from build123d import *

# Parameters (mm, degrees)
SKETCH1_W           = 79.816604327
SKETCH1_H           = 61.580684207
BOSS_EXTRUDE1_DEPTH = 20
CUT_EXTRUDE1_START  = -18.943875
SKETCH3_R           = 4
CUT_EXTRUDE1_DEPTH  = 80.816604514


with BuildPart() as part:
    # Sketch1 → Boss-Extrude1 (new body)
    with BuildSketch(Plane.XY):
        with Locations((-58.852177351, -19.652156424)):
            Rectangle(SKETCH1_W, SKETCH1_H)
    extrude(amount=BOSS_EXTRUDE1_DEPTH)

    # Sketch3 → Cut-Extrude1 (cut, through all)
    with BuildSketch(Plane(origin=(0, 0, 0), x_dir=(0, 0, -1), z_dir=(1, 0, 0)).offset(CUT_EXTRUDE1_START)):
        with Locations((-10, -5.101602078)):
            Circle(SKETCH3_R)
    extrude(amount=-CUT_EXTRUDE1_DEPTH, mode=Mode.SUBTRACT)


solid = part.part
Design review of the part built by this model. Coordinates are the model's own, in mm. Give positions to 0.01 mm unless a question says otherwise; leave off trailing zeros. Write each loop counter-clockwise with the first axis right and the second up, starting at its lowest first coordinate (ties: lowest second). Pieces come first, ordered by that corner, then holes. Notation, with made-up numbers: M -36,21 L -3,21 A12 cw -3,29 Z; hole C -24.75,-16.75 d11. An arc over 180 degrees is marked long. Return JSON: item names as keys, results as strings. Group by question number.
Item 1: Take a section at A-A (z = 10). Give the boundary of the cut face in (x, y), plus the area to 3 significant figures.
Item 2: Take a section at B-B (x = -44). Give the boundary of the cut face in (y, z), plus the area to 3 significant figures.
Item 3: The part is to be moulded in two halves that separate along Y. For faces 1 (the flat face through (-59, -19, 20)), 2 (the flat face through (-59, -50.442, 10)), 3 (the cylindrical face through (-58.3, -9, 10.9)), say which applies: pulls with the +Y half, pulls with the -Y half, needs draft (parallel to the pull), parting line crosses it, or undercut.
Item 4: Wall thickness on line 1 along Y through (x, z) = (-64, 10); line 2 along Y through (x, z) = (-86, 9.25); line 3 along Z through (x, y) = (-93, -7): over which ranges is each line inside the solid? List them lowest first.
Return value:
{
 "1": {"outline": "M -98.76,-50.44 L -18.94,-50.44 L -18.94,-9.1 L -98.76,-9.1 Z; M -98.76,-1.1 L -18.94,-1.1 L -18.94,11.14 L -98.76,11.14 Z", "area": "4,280 mm2"},
 "2": {"outline": "M -50.44,0 L 11.14,0 L 11.14,20 L -50.44,20 Z; hole C -5.1,10 d8", "area": "1,180 mm2"},
 "3": {"face 1": "needs draft", "face 2": "pulls with the -Y half", "face 3": "undercut"},
 "4": {"line 1": "y = -50.44 to -9.1, -1.1 to 11.14", "line 2": "y = -50.44 to -9.03, -1.17 to 11.14", "line 3": "z = 0 to 6.48, 13.52 to 20"}
}
